Autodesk Inventor part; units mm, degrees
ref_plane "Start Plane" through (0, 0, 15) normal (0, 0, 1) x (1, 0, 0)
ref_plane "End Plane" through (0, 0, 1386) normal (0, 0, 1) x (1, 0, 0)
ref_plane "Work Plane4" through (9, -520, 15) normal (0, 0, -1) x (-1, 0, 0)
ref_plane "Start Plane" through (0, 0, 15) normal (0, 0, 1) x (1, 0, 0)
ref_plane "End Plane" through (0, 0, 1386) normal (0, 0, 1) x (1, 0, 0)
sketch "Sketch" plane through (0, 0, 0) normal (0, 0, 1) x (1, 0, 0)
  line L0 (-15, -9) -> (-15, 9)
  line L1 (-9, 15) -> (9, 15)
  line L2 (15, 9) -> (15, -9)
  line L3 (9, -15) -> (-9, -15)
  arc A0 (-15, -9) -> (-9, -15) centre (-9, -9) ccw
  arc A1 (-9, 15) -> (-15, 9) centre (-9, 9) ccw
  arc A2 (15, 9) -> (9, 15) centre (9, 9) ccw
  arc A3 (9, -15) -> (15, -9) centre (9, -9) ccw
  arc A4 (-9, 12) -> (-12, 9) centre (-9, 9) ccw
  line L4 (-9, 12) -> (9, 12)
  arc A5 (12, 9) -> (9, 12) centre (9, 9) ccw
  line L5 (12, 9) -> (12, -9)
  arc A6 (9, -12) -> (12, -9) centre (9, -9) ccw
  line L6 (9, -12) -> (-9, -12)
  arc A7 (-12, -9) -> (-9, -12) centre (-9, -9) ccw
  line L7 (-12, -9) -> (-12, 9)
  line L8 (0, 22.7397) -> (0, -22.7397) construction
  line L9 (-22.7397, 0) -> (22.7397, 0) construction
  dimension "d7" = 6
  dimension "d10" = 30
  dimension "d11" = 30
  dimension "d12" = 3
  dimension "d15" = 15
  dimension "d16" = 15
extrude "Body" add sketch "Sketch" along normal up to surface (1371 mm away) from surface at 15
sketch "Sketch3" plane through (0, 0, 0) normal (0, 0, 1) x (1, 0, 0)
  line L0 (0, 0) -> (10, 0)
ref_plane "Work Plane3" through (0, 0, 0) normal (0, -1, 0) x (1, 0, 0)
ref_plane "Work Plane4" through (9, -520, 15) normal (0, 0, -1) x (-1, 0, 0)
split "Split1" plane through (9, -520, 15) removes the side toward (0, 0, -1)
ref_plane "Work Plane5" through (9, 230, 1386) normal (0, 0, 1) x (1, 0, 0)
split "Split2" plane through (9, 230, 1386) removes the side toward (0, 0, 1)
sketch "Sketch4" plane through (0, 0, 0) normal (0, -1, 0) x (1, 0, 0)
  line L0 (-2, 15) -> (12, 15)
  line L1 (-2, 1386) -> (12, 1386)
  dimension "d18" = 1371
equation "\"d7\" = G_IR"
equation "\"d10\" = G_H"
equation "\"d11\" = G_W"
equation "\"d12\" = G_T"
equation "\"d15\" = 0.5 * d10"
equation "\"d16\" = 0.5 * d11"
equation "\"d3\" = G_L"
equation "\"G_W\" = 30"
equation "\"G_H\" = 30"
equation "\"G_T\" = 3"
equation "\"G_IR\" = 6"
equation "\"G_L\" = d18"
equation "\"G_OFFSET_START\" = -15"
equation "\"G_OFFSET_END\" = -15"
equation "\"d13\" = -G_OFFSET_START"
equation "\"d14\" = G_OFFSET_END + B_L"
equation "\"B_L\" = 1401"
properties part number "DIN EN 10219-2 - 30 x 30 x 3  - 1371" material "Steel, Mild"
Here's how the part is built. I have some questions about the finished solid (model axes, mm). Round coordinates to 2 decimals unless told otherwise and drop trailing zeros. Order: outer loops, then holes, each group sorted by start corner. A loop starts at its lowest first (then second) coordinate and runs counter-clockwise, first axis right, second up. Notation, with made-up numbers: M 70,-30.5 L 108,-30.5 A24 cw 108,-8.5 Z; hole C 31.25,-20.5 d9. An arc over 180 degrees is marked long. Return JSON: item names as keys, results as strings. Group by question number.
1. If we section it at C-C on z = 176: List the corners of the cut face in (x, y) for me.
2. If we section it at A-A on y = -2.25: List the corners of the cut face in (x, z) for me.
3. Please list where these lines run through material, in increasing order: probe 1 along Y at (x, z) = (10, 805); probe 2 along Y at (x, z) = (5, 918.5); probe 3 along X at (y, z) = (10.25, 503).
4. I'm going to push flat-ended pins straight in: pin 1 Ø2 at (x, y) = (2.5, 10.5) entering from -Z; pin 2 Ø3 at (y, z) = (-12, 288.5) entering from -X. Where does each tip first touch, or does it pass through?
Reply:
{
 "1": {"outline": "M -15,-9 A6 ccw -9,-15 L 9,-15 A6 ccw 15,-9 L 15,9 A6 ccw 9,15 L -9,15 A6 ccw -15,9 Z; hole M -12,-9 A3 ccw -9,-12 L 9,-12 A3 ccw 12,-9 L 12,9 A3 ccw 9,12 L -9,12 A3 ccw -12,9 Z"},
 "2": {"outline": "M -15,15 L -12,15 L -12,1386 L -15,1386 Z; M 12,15 L 15,15 L 15,1386 L 12,1386 Z"},
 "3": {"probe 1": "-14.92 to -11.83, 11.83 to 14.92", "probe 2": "-15 to -12, 12 to 15", "probe 3": "-14.87 to -11.73, 11.73 to 14.87"},
 "4": {"pin 1": "through", "pin 2": "x = -14.81"}
}
